```python
from build123d import *

# Parameters (mm, degrees)
F1_DEPTH = 88.9
F2_W     = 89.568419
F2_H     = 63.5
F3_DEPTH = 215.9
F4_R     = 16.129
F5_DEPTH = 16.764


with BuildPart() as f1:
    # F0 (on Top) → F1 (new body)
    with BuildSketch(Plane.XY):
        Polygon((44.45, 25.663219), (-44.45, 25.663219), (0, -51.326439), align=None)
    extrude(amount=F1_DEPTH)

    # F2 (on Top) → F3 (intersect)
    with BuildSketch(Plane.XY):
        with Locations((-0.249351, -5.168639)):
            Rectangle(F2_W, F2_H)
    extrude(amount=F3_DEPTH, mode=Mode.INTERSECT)

    # F4 (on Top) → F5 (cut)
    with BuildSketch(Plane.XY):
        Circle(F4_R)
    extrude(amount=F5_DEPTH, mode=Mode.SUBTRACT)


solid = f1.part
```
Check sheet for the modelled part. Datum: model origin and axes. Units: mm. A direction names the side the tool comes from. Coordinates: 2 decimals unless noted, no trailing zeros. Write each loop counter-clockwise with the first axis right and the second up, starting at its lowest first coordinate (ties: lowest second). Pieces come first, ordered by that corner, then holes. Notation, with made-up numbers: M 82,18 L 103,18 A16 cw 103,35 Z; hole C 11.25,83.25 d5. An arc over 180 degrees is marked long. Write item = value, one per line. Start each with the question number.
1. Sectioned sample at D-D (z = 78). Record the cut outline in (x, y).
2. Sectioned sample at B-B (z = 7). Record the cut outline in (x, y).
3. Thickness scan on probe 1 along Y at (x, z) = (0, 12.5); probe 2 along Z at (x, y) = (6, -8); probe 3 along X at (y, z) = (-3, 13.5). Record the ranges inside material, lowest first.
4. Sectioned sample at A-A (x = 0). Record the cut outline in (y, z), then the cut area to 3 significant figures.
5. Tool access check on faces 4 (the flat face through (0, 0, 16.764)), 5 (the flat face through (-11, 16, 0)). Record the directions out of +Z, -Z, +X, -X, +Y, -Y that give a thin tool (end or side, any length) a straight path to the whole face; none if there is none.
6. Go/stop test with flat-tipped pins: pin 1 (3 mm diameter, centred on y = 12, z = 46, fed in from -X); pin 2 (8 mm diameter, centred on y = -15.5, z = 18, fed in from -X); pin 3 (9.5 mm diameter, centred on x = 2.5, y = -5.5, fed in from -Z). Record where each tip stops, or that it passes through.
7. Sectioned sample at C-C (y = 0). Record the cut outline in (x, z), then the cut area to 3 significant figures.
8. Mould release check, pull along X, two halves, no side actions. Record for faces 1 (the flat face through (-26.637, -5.19, 43.828)), 2 (the cylindrical face through (15.4, 4.8, 8.3)), 3 (the flat face through (-1, 2, 88.9)): pulls with the +X half, pulls with the -X half, needs draft (parallel to the pull), parting line crosses it, or undercut.
The answers:
q1.outline = M -44.45,25.66 L -8.32,-36.92 L 8.32,-36.92 L 44.45,25.66 Z
q2.outline = M -44.45,25.66 L -8.32,-36.92 L 8.32,-36.92 L 44.45,25.66 Z; hole C 0,0 d32.26
q3.probe_1 = -36.92 to -16.13, 16.13 to 25.66
q3.probe_2 = 16.76 to 88.9
q3.probe_3 = -27.9 to -15.85, 15.85 to 27.9
q4.outline = M -36.92,0 L -16.13,0 L -16.13,16.76 L 16.13,16.76 L 16.13,0 L 25.66,0 L 25.66,88.9 L -36.92,88.9 Z
q4.area = 5,020 mm²
q5.face_4 = -Z
q5.face_5 = -Z, +X, -X, +Y, -Y
q6.pin_1 = -37.43
q6.pin_2 = -22.99
q6.pin_3 = 16.76
q7.outline = M -29.63,0 L -16.13,0 L -16.13,16.76 L 16.13,16.76 L 16.13,0 L 29.63,0 L 29.63,88.9 L -29.63,88.9 Z
q7.area = 4,730 mm²
q8.face_1 = pulls with the -X half
q8.face_2 = undercut
q8.face_3 = needs draft
